CAD build for the part. Positions are in the model's coordinates, mm. A direction names the side the tool comes from. Give positions to 0.01 mm unless a question says otherwise; leave off trailing zeros. Loops run counter-clockwise (first coordinate to the right, second up) from the corner with the lowest first, then second, coordinate; pieces in that order, holes last. Notation, with made-up numbers: (58, -16.5) - (92, -16.5) arc R11 ccw to (92, -2.5) - close; hole circle Ø8 at (-37, 85.5). An arc over 180 degrees is marked (long way). Return JSON: item names as keys, results as strings.
from build123d import *

# Parameters (mm, degrees)
ESQUISSE1_R        = 1.5
BOSS_EXTRU_1_DEPTH = 5
CONG_1_R           = 17
CONG_2_R           = 10


with BuildPart() as part:
    # Esquisse1 → Boss.-Extru.1 (new body)
    with BuildSketch(Plane.XY):
        Polygon((0, 0), (25, 0), (32, 0), (32, 61), (31.250785563, 61), (27.30740989, 54.169872981), (22.977282871, 56.669872981), (25.477282871, 61), (15, 61), (0, 61), align=None)
        with Locations((10, 54.5)):
            Circle(ESQUISSE1_R, mode=Mode.SUBTRACT)
        with Locations((20, 6.5)):
            Circle(ESQUISSE1_R, mode=Mode.SUBTRACT)
        with Locations(Location((10, 6.5, 0), (0, 0, 180))):
            Circle(ESQUISSE1_R, mode=Mode.SUBTRACT)
        Polygon((14, 51), (5, 51), (5, 10), (14, 10), (14, 7), (16, 7), (16, 10), (25, 10), (25, 51), (16, 51), (16, 54), (14, 54), align=None, mode=Mode.SUBTRACT)
    extrude(amount=BOSS_EXTRU_1_DEPTH)

    # Congé1
    cong_1_edges = [part.edges().sort_by_distance(p)[0] for p in [
        (0, 61, 2.5),
    ]]
    fillet(cong_1_edges, radius=CONG_1_R)

    # Congé2
    cong_2_edges = [part.edges().sort_by_distance(p)[0] for p in [
        (0, 0, 2.5),
    ]]
    fillet(cong_2_edges, radius=CONG_2_R)


solid = part.part
1. Cut at A-A, the plane x = 20. Write the cut outline in (y, z).
Values follow:
{"outline": "(0, 0) - (5, 0) - (5, 5) - (0, 5) - close; (8, 0) - (10, 0) - (10, 5) - (8, 5) - close; (51, 0) - (61, 0) - (61, 5) - (51, 5) - close"}
2. Cut at B-B, the plane y = 31.5. Write the cut outline in (x, z), plus the area to 3 significant figures.
Values follow:
{"outline": "(0, 0) - (5, 0) - (5, 5) - (0, 5) - close; (25, 0) - (32, 0) - (32, 5) - (25, 5) - close", "area": "60.0 mm²"}
3. Cut at D-D, the plane y = 48.5. Write the cut outline in (x, z), plus the area to 3 significant figures.
Values follow:
{"outline": "(0.61, 0) - (5, 0) - (5, 5) - (0.61, 5) - close; (25, 0) - (32, 0) - (32, 5) - (25, 5) - close", "area": "57.0 mm²"}
4. Pull direction Y, two halves, no side cores. Call faces 1 (the face through (29.307, 57.633, 2.465)), 2 (the face through (11.2, 7.4, 2.5)), 3 (the face through (26, 31, 0)): +Y half, -Y half, draft (parallel to the pull), parting line (faces both ways), or undercut.
Values follow:
{"face 1": "+Y half", "face 2": "undercut", "face 3": "draft"}
5. Which spindle directions (+Z, -Z, +X, -X, +Y, -Y) get a long thin tool onto all of the face, cutting with end or side? Do faces 4 (the face through (21, 61, 2)), 5 (the face through (16, 8, 2)). Say none if no direction does.
Values follow:
{"face 4": "+Z, -Z, +X, -X, +Y", "face 5": "+Z, -Z"}
6. Cut at C-C, the plane z = 4.3. Write the cut outline in (x, y), plus the area to 3 significant figures.
Values follow:
{"outline": "(0, 10) arc R10 ccw to (10, 0) - (32, 0) - (32, 61) - (31.25, 61) - (27.31, 54.17) - (22.98, 56.67) - (25.48, 61) - (17, 61) arc R17 ccw to (0, 44) - close; hole (5, 10) - (14, 10) - (14, 7) - (16, 7) - (16, 10) - (25, 10) - (25, 51) - (16, 51) - (16, 54) - (14, 54) - (14, 51) - (5, 51) - close; hole circle Ø3 at (10, 6.5); hole circle Ø3 at (10, 54.5); hole circle Ø3 at (20, 6.5)", "area": "983 mm²"}
7. Drop flat-ended pins along their axis: P1, Ø3.5, axis at x = 10, y = 6.5, coming from the -Z side; P2, Ø12, axis at x = 17, y = 27.5, coming from the -Z side; P3, Ø1.5, axis at y = 9, z = 2, coming from the -X side; P4, Ø1, axis at x = 15, z = 3, coming from the +Y side. Give the stop position or say it passes through.
Values follow:
{"P1": "stops at z = 0", "P2": "passes through", "P3": "stops at x = 0", "P4": "stops at y = 60.93"}
8. Drill centre lines: probe 1 along X at (y, z) = (11, 2.05); probe 2 along Y at (x, z) = (10, 1.3); probe 3 along Y at (x, z) = (18, 0.35). Where is each one in solid material? Low to high.
Values follow:
{"probe 1": "x = 0 to 5, 25 to 32", "probe 2": "y = 0 to 5, 8 to 10, 51 to 53, 56 to 59.49", "probe 3": "y = 0 to 10, 51 to 61"}
